Part model, mm, in its own coordinate system. Face numbers are marked on the shaded views. A direction names the side the tool comes from. Round coordinates to 2 decimals unless told otherwise and drop trailing zeros. Write each loop counter-clockwise with the first axis right and the second up, starting at its lowest first coordinate (ties: lowest second). Pieces come first, ordered by that corner, then holes. Notation, with made-up numbers: M 9.5,19 L 22.5,19 A17 ccw 22.5,37 Z; hole C -22,-22.5 d3. An arc over 180 degrees is marked long. Answer as a JSON object with one key per item and string values. Group by question number.
1. Band-saw the part on D-D, the plane y = 5. Write the cut outline in (x, z), plus the area to 3 significant figures.
2. Drill centre lines: line 1 (X direction, y = -0.5, z = 12); line 2 (Z direction, x = -27.5, y = 2.5); line 3 (X direction, y = 9, z = 21.5). Where is each one in solid material? Low to high. Write a range as from..to.
3. Drop a flat-ended pin along its axis: pin 1 (2 mm diameter, centred on x = -31, z = -1, fed in from +Y). Give the stop position or say it passes through.
4. Two-plate mould, pull along Y, no slides. Class the marked faces 1, 2 and 3: +Y half, -Y half, draft (parallel to the pull), parting line (faces both ways), or undercut.
5. Which spindle directions (+Z, -Z, +X, -X, +Y, -Y) get a long thin tool onto all of the face, cutting with end or side? Do the marked faces 4, 5 and 6. Say none if no direction does.
6. Band-saw the part on A-A, the plane z = -4. Write the cut outline in (x, y) (1 decimal).
7. Band-saw the part on B-B, the plane y = 0. Write the cut outline in (x, z).
8. Band-saw the part on C-C, the plane x = -6. Write the cut outline in (y, z), plus the area to 3 significant figures.
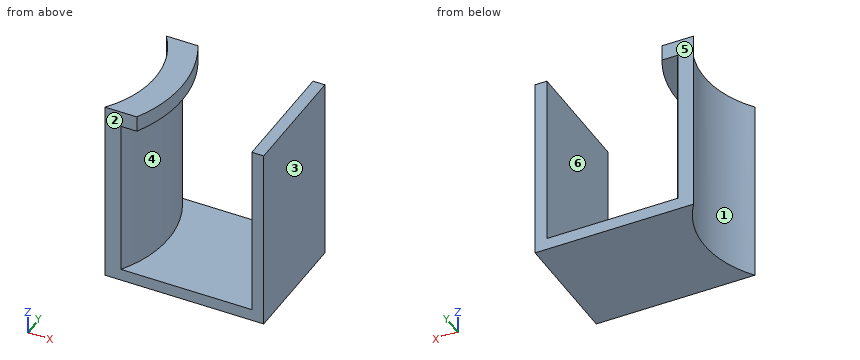
Autodesk Inventor part; units mm, degrees
ref_plane "YZ Plane" through (0, 0, 0) normal (1, 0, 0) x (0, 1, 0)
ref_plane "XZ Plane" through (0, 0, 0) normal (0, 1, 0) x (-1, 0, 0)
ref_plane "XY Plane" through (0, 0, 0) normal (0, 0, 1) x (1, 0, 0)
sketch "Sketch1" plane through (0, 0, 0) normal (1, 0, 0) x (0, 1, 0)
  line L0 (-15, -15) -> (15, -15)
  line L1 (15, -15) -> (15, 15)
  line L2 (15, 15) -> (-15, 15)
  line L3 (-15, 15) -> (-15, -15)
  line L4 (-15, -15) -> (15, 15) construction
  line L5 (15, -15) -> (-15, 15) construction
  point P0 (0, 0)
  dimension "d0" = 30
  dimension "d1" = 30
extrude "Extrusion1" add sketch "Sketch1" along normal blind 3
sketch "Sketch2" plane through (0, -15, -15) normal (0, 0, -1) x (-1, 0, 0)
  line L0 (0, 30) -> (-3, 30)
  line L1 (-3, 30) -> (37, 30)
  line L2 (37, 30) -> (37, 0)
  line L3 (37, 0) -> (-3, 0)
  line L4 (-3, 0) -> (-3, 30)
  point P0 (0, 15)
  dimension "d4" = 40
  dimension "d5" = 30
extrude "Extrusion2" add sketch "Sketch2" along normal blind 3
sketch "Sketch3" plane through (0, -15, -15) normal (0, 0, 1) x (1, 0, 0)
  line L0 (0, 0) -> (-37, 0)
  line L1 (-37, 0) -> (-37, 30)
  arc A0 (-37, 0) -> (-37, 30) centre (-57.325, 15) ccw
  point P0 (0, 15)
extrude "Extrusion3" cut sketch "Sketch3" against normal blind 3
sketch "Sketch4" plane through (0, -15, -15) normal (0, 0, 1) x (1, 0, 0)
  line L0 (-37, 30) -> (0, 30)
  arc A0 (-37, 0) -> (-37, 30) centre (-57.325, 15) ccw
  line L1 (-33.6755, 30) -> (-37, 30)
  point P0 (0, 15)
sketch "Sketch5" plane through (0, -15, -15) normal (0, 0, 1) x (1, 0, 0)
  arc A0 (-37, 0) -> (-37, 30) centre (-57.325, 15) ccw
  line L0 (-37, 30) -> (-33, 30)
  line L1 (-37, 30) -> (0, 30)
  line L2 (0, 0) -> (-37, 0)
  arc A1 (-33, 0) -> (-33, 30) centre (-57.325, 15) ccw
  line L3 (-33, 0) -> (-37, 0)
  arc A2 (-37, 0) -> (-37, 30) centre (-57.325, 15) ccw
  point P0 (0, 15)
  dimension "d10" = 4
extrude "Extrusion4" add sketch "Sketch5" along normal blind 40
sketch "Sketch6" plane through (0, -15, 25) normal (0, 0, 1) x (1, 0, 0)
  line L0 (-33, 30) -> (-37, 30)
  line L1 (-37, 30) -> (-29, 30)
  arc A0 (-37, 0) -> (-37, 30) centre (-57.325, 15) ccw
  line L2 (-37, 0) -> (-29, 0)
  arc A1 (-29, 0) -> (-29, 30) centre (-57.325, 15) ccw
  arc A2 (-37, 0) -> (-37, 30) centre (-57.325, 15) ccw
  point P0 (0, 15)
  dimension "d13" = 8
extrude "Extrusion5" add sketch "Sketch6" along normal blind 4
sketch "Sketch7" plane through (0, -15, 15) normal (0, -1, 0) x (1, 0, 0)
  point P0 (0, -15)
sketch "Sketch8" plane through (0, -15, 15) normal (0, 0, 1) x (1, 0, 0)
  point P0 (0, 15)
sketch "Sketch9" plane through (0, -15, 15) normal (0, -1, 0) x (1, 0, 0)
  line L0 (3, 0) -> (3, -33)
  line L1 (3, 0) -> (3, 14)
  line L2 (3, 14) -> (0, 14)
  line L3 (0, 0) -> (3, 0)
  line L4 (0, 14) -> (0, 0)
  line L5 (0, 0) -> (3, 0)
  point P0 (0, -15)
  dimension "d16" = 14
extrude "Extrusion6" add sketch "Sketch9" against normal blind 30
sketch "Sketch10" plane through (0, 0, 0) normal (-1, 0, 0) x (0, 0, 1)
  point P0 (0, 0)
properties part number "headphones_hookl"
Worked answers:
{
 "1": {"outline": "M -32.56,-18 L 3,-18 L 3,29 L 0,29 L 0,-15 L -29.19,-15 L -29.19,25 L -25.67,25 L -25.67,29 L -32.56,29 Z", "area": "401 mm^2"},
 "2": {"line 1": "x = -32.07..-28.75, 0..3", "line 2": "z = -18..-15, 25..29", "line 3": "x = -33.72..-30.2, 0..3"},
 "3": {"pin 1": "stops at y = 13.24"},
 "4": {"face 1": "undercut", "face 2": "-Y half", "face 3": "draft"},
 "5": {"face 4": "none", "face 5": "+Z, -Z, +X, -X, +Y", "face 6": "+Z, +Y, -Y"},
 "6": {"outline": "M -37,-15 L -33,-15 A28.6 ccw -33,15 L -37,15 A25.3 cw Z; M 0,-15 L 3,-15 L 3,15 L 0,15 Z"},
 "7": {"outline": "M -32.06,-18 L 3,-18 L 3,29 L 0,29 L 0,-15 L -28.75,-15 L -28.75,25 L -25.27,25 L -25.27,29 L -32.06,29 Z"},
 "8": {"outline": "M -15,-18 L 15,-18 L 15,-15 L -15,-15 Z", "area": "90.0 mm^2"}
}
